Part model, mm, in its own coordinate system. Face numbers are marked on the shaded views. Coordinates: 2 decimals unless noted, no trailing zeros. Loops run counter-clockwise (first coordinate to the right, second up) from the corner with the lowest first, then second, coordinate; pieces in that order, holes last. Notation, with made-up numbers: (65, 30) - (115, 30) arc R24 cw to (115, 55) - close; hole circle Ø6 at (47.5, 87.5). An arc over 180 degrees is marked (long way). Use a Markdown table: item, result. Add a question column.
1. Drop flat-ended pins along their axis: pin 1 (12 mm diameter, centred on x = -38, y = -2.5, fed in from -Z); pin 2 (2 mm diameter, centred on x = 113, y = -9, fed in from -Z); pin 3 (4 mm diameter, centred on x = 94.5, z = -5.5, fed in from -Y). Give the stop position or say it passes through.
2. Band-saw the part on A-A, the plane y = 6.5. Give the cut face in (x, z), plus the area to 3 significant figures.
3. Pull direction Y, two halves, no side cores. Call the marked faces 1, 2, 3 and 4: pulls with the +Y half, pulls with the -Y half, needs draft (parallel to the pull), parting line crosses it, or undercut.
4. Band-saw the part on C-C, the plane y = -13.5. Give the cut face in (x, z).
5. Band-saw the part on B-B, the plane x = 178. Give the cut face in (y, z), plus the area to 3 significant figures.
6. Wall check: probe 1 along Z at (x, y) = (-54, 9); probe 2 along Z at (x, y) = (-134.5, 1). Give the ranges that are in metal, low to high. Write a range as [from, to].
from build123d import *

# Parameters (mm, degrees)
EXTRUSION1_DEPTH = 1.5
ESQUISSE3_W      = 400
ESQUISSE3_H      = 46
EXTRUSION2_DEPTH = 130
ESQUISSE4_W      = 400
ESQUISSE4_H      = 15
EXTRUSION3_DEPTH = 145


with BuildPart() as part:
    # Esquisse2 → Extrusion1 (new body)
    with BuildSketch(Plane.XY):
        with BuildLine():
            Line((238, -21), (70.5, -21))
            Line((70.5, -21), (70.5, -8))
            ThreePointArc((70.5, -8), (71.085786438, -6.585786438), (72.5, -6))
            Line((72.5, -6), (83, -6))
            ThreePointArc((83, -6), (95.5, 6.5), (83, 19))
            Line((83, 19), (-70.25, 19))
            ThreePointArc((-70.25, 19), (-82.75, 6.5), (-70.25, -6))
            Line((-70.25, -6), (-61.5, -6))
            ThreePointArc((-61.5, -6), (-60.085786438, -6.585786438), (-59.5, -8))
            Line((-59.5, -8), (-59.5, -21))
            Line((-59.5, -21), (-162, -21))
            Line((-162, -21), (-162, 25))
            Line((-162, 25), (238, 25))
            Line((238, 25), (238, -21))
        make_face()
    extrude(amount=-EXTRUSION1_DEPTH)

    # Esquisse3 → Extrusion2 (add)
    with BuildSketch(Plane.XY):
        with Locations((38, 2)):
            Rectangle(ESQUISSE3_W, ESQUISSE3_H)
    extrude(amount=EXTRUSION2_DEPTH)

    # Esquisse4 → Extrusion3 (add)
    with BuildSketch(Plane.XY.offset(130)):
        with Locations((38, 32.5)):
            Rectangle(ESQUISSE4_W, ESQUISSE4_H)
    extrude(amount=-EXTRUSION3_DEPTH)


solid = part.part
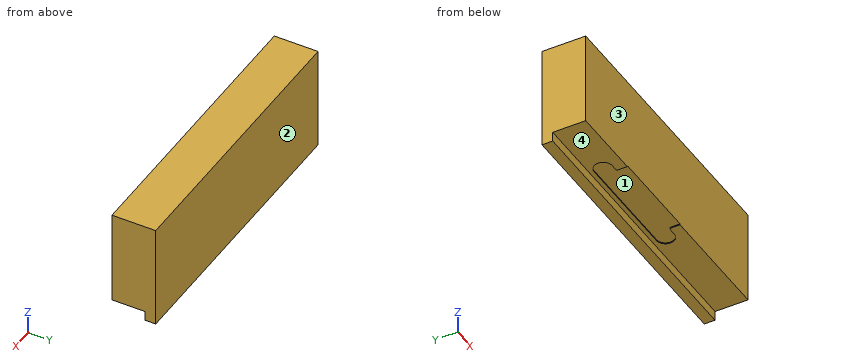
Geometry check:
| question | item | result |
|---|---|---|
| 1 | pin 1 | stops at z = 0 |
| 1 | pin 2 | stops at z = -1.5 |
| 1 | pin 3 | stops at y = 25 |
| 2 | outline | (-162, -1.5) - (-82.75, -1.5) - (-82.75, 0) - (95.5, 0) - (95.5, -1.5) - (238, -1.5) - (238, 130) - (-162, 130) - close |
| 2 | area | 52,300 mm^2 |
| 3 | face 1 | undercut |
| 3 | face 2 | pulls with the +Y half |
| 3 | face 3 | pulls with the -Y half |
| 3 | face 4 | needs draft |
| 4 | outline | (-162, -1.5) - (-59.5, -1.5) - (-59.5, 0) - (70.5, 0) - (70.5, -1.5) - (238, -1.5) - (238, 130) - (-162, 130) - close |
| 5 | outline | (-21, -1.5) - (25, -1.5) - (25, -15) - (40, -15) - (40, 130) - (-21, 130) - close |
| 5 | area | 8,220 mm^2 |
| 6 | probe 1 | z = [0, 130] |
| 6 | probe 2 | z = [-1.5, 130] |
